Source: CAD feature listing. Evaluate the final solid. Frame: model axes, mm. A direction names the side the tool comes from. Coordinates: 2 decimals unless noted, no trailing zeros.
```python
from build123d import *

# Parameters (mm, degrees)
F1_DEPTH = 127
F1_TAPER = -10


with BuildPart() as f1:
    # F0 (on Front) → F1 (new body, symmetric)
    with BuildSketch(Plane.XZ):
        with BuildLine():
            Line((9.4366056551, 31.9971223519), (-29.0780882326, 25.645936495))
            ThreePointArc((-29.0780882326, 25.645936495), (-41.424375402, 16.4380068606), (-41.0428613167, 1.0408895322))
            Line((-41.0428613167, 1.0408895322), (-22.2548710668, -33.1750516271))
            ThreePointArc((-22.2548710668, -33.1750516271), (56.5854242226, -31.2215247106), (9.4366056551, 31.9971223519))
        make_face()
    extrude(amount=F1_DEPTH, both=True, taper=F1_TAPER)


solid = f1.part
```
Q1. Set-up query: faces 4 (the flat face through (-11.4, -64.39, 40.07)), 5 (the flat face through (-41.732, -64.389, -21.292)), 6 (the conical face through (66.026, -64.389, -37.71)). Return all of +Z, -Z, +X, -X, +Y, -Y with unobstructed straight access to the full face (end or side cutting, diameter ignored); none if empty.
Solutions:
face 4: +Z, -X
face 5: -Z, -X
face 6: none
Q2. Pin query (flat end, axial travel): P1, Ø3, axis at y = 4, z = -31.5, coming from the -X side; P2, Ø12, axis at x = 32.5, y = -9.5, coming from the +Z side; P3, Ø4, axis at y = 4, z = -35, coming from the -X side. Return the tip coordinate at first contact, or that it passes through.
Solutions:
P1: stops at x = -24.86
P2: stops at z = 33.58
P3: stops at x = -23.23
Q3. Pull-direction query (Y, two-part tool) for faces 1 (the flat face through (10, -127, -14)), 2 (the conical face through (66.026, 64.389, -37.71)), 3 (the flat face through (10, 127, -14)); classes: pulls with the +Y half, pulls with the -Y half, needs draft (parallel to the pull), parting line crosses it, or undercut.
Solutions:
face 1: pulls with the -Y half
face 2: undercut
face 3: pulls with the +Y half
Q4. Material intervals for line 1 along Z through (x, y) = (38, 106.5); line 2 along Z through (x, y) = (-31.5, 74); line 3 along X through (y, z) = (58.5, -8), sorted ascending.
Solutions:
line 1: z = -71.27 to 47.65
line 2: z = -43.12 to 38.47
line 3: x = -47.85 to 71.24
